Work out the finished part from the listing and answer in its coordinate system (mm). A direction names the side the tool comes from. Coordinates: 2 decimals unless noted, no trailing zeros. Order: outer loops, then holes, each group sorted by start corner. A loop starts at its lowest first (then second) coordinate and runs counter-clockwise, first axis right, second up. Notation, with made-up numbers: M 3,35.5 L 16,35.5 A8 cw 16,44.5 Z; hole C 80,57.25 d9. An arc over 180 degrees is marked long. Use a Markdown table: item, result.
from build123d import *

# Parameters (mm, degrees)
F0_W     = 5
F0_H     = 15
F1_DEPTH = 10
F3_DEPTH = 20.001
F4_W     = 10
F4_H     = 5
F5_DEPTH = 30.001


with BuildPart() as f1:
    # F0 (on Top) → F1 (new body, symmetric)
    with BuildSketch(Plane.XY):
        Polygon((0, 20), (0, 0), (20, 0), (20, 5), (25, 5), (25, 20), align=None)
        with Locations((27.5, 12.5)):
            Rectangle(F0_W, F0_H)
    extrude(amount=F1_DEPTH, both=True)

    # F2 (on Front) → F3 (cut, through all)
    with BuildSketch(Plane.XZ):
        with BuildLine():
            Line((0, 10), (0, 2.5))
            ThreePointArc((0, 2.5), (3.75, 7.916667), (10, 10))
            Line((10, 10), (0, 10))
        make_face()
        with BuildLine():
            ThreePointArc((10, -10), (3.75, -7.916667), (0, -2.5))
            Line((0, -2.5), (0, -10))
            Line((0, -10), (10, -10))
        make_face()
        Polygon((25, 10), (30, 5), (30, 10), align=None)
        Polygon((30, -10), (30, -5), (25, -10), align=None)
        with BuildLine():
            ThreePointArc((14.330127, -2.5), (14.829629, -1.294095), (15, 0))
            ThreePointArc((15, 0), (14.829629, 1.294095), (14.330127, 2.5))
            ThreePointArc((14.330127, 2.5), (10, 5), (5.669873, 2.5))
            ThreePointArc((5.669873, 2.5), (5, 0), (5.669873, -2.5))
            ThreePointArc((5.669873, -2.5), (10, -5), (14.330127, -2.5))
        make_face()
    extrude(amount=-F3_DEPTH, mode=Mode.SUBTRACT)

    # F4 (on Right) → F5 (cut, through all)
    with BuildSketch(Plane.YZ):
        with Locations((5, 0)):
            Rectangle(F4_W, F4_H)
    extrude(amount=F5_DEPTH, mode=Mode.SUBTRACT)


solid = f1.part
(1) Straight lines are drawn through the part: L1, parallel to Z at x = 24.5, y = 5.5; L2, parallel to Y at x = 25.5, z = 6.75; L3, parallel to Y at x = 17, z = 0. For each, find the intervals that lie inside material, in ascending order.
Conclusion:
| item | result |
|---|---|
| L1 | -10 to -2.5, 2.5 to 10 |
| L2 | 5 to 20 |
| L3 | 10 to 20 |
(2) A cutting plane is placed at A-A (y = 3). Determine the outline of the cut face in (x, z), then the cut area to 3 significant figures.
Conclusion:
| item | result |
|---|---|
| outline | M 0,-2.5 A10.42 ccw 10,-10 L 20,-10 L 20,-2.5 L 14.33,-2.5 A5 cw 5.67,-2.5 Z; M 0,2.5 L 5.67,2.5 A5 cw 14.33,2.5 L 20,2.5 L 20,10 L 10,10 A10.42 ccw Z |
| area | 230 mm2 |
(3) A cutting plane is placed at D-D (z = 4). Determine the outline of the cut face in (x, y), then the cut area to 3 significant figures.
Conclusion:
| item | result |
|---|---|
| outline | M 0.57,0 L 7,0 L 7,20 L 0.57,20 Z; M 13,0 L 20,0 L 20,5 L 30,5 L 30,20 L 13,20 Z |
| area | 419 mm2 |
(4) Determine the mould class of faces 4 (the flat face through (17, 10, -10)), 5 (the flat face through (22, 10, 0)), 6 (the flat face through (12, 0, 6)) for opening direction Z: pulls with the +Z half, pulls with the -Z half, needs draft (parallel to the pull), parting line crosses it, or undercut.
Conclusion:
| item | result |
|---|---|
| face 4 | pulls with the -Z half |
| face 5 | undercut |
| face 6 | needs draft |
(5) A cutting plane is placed at C-C (x = 7.5). Determine the outline of the cut face in (y, z).
Conclusion:
| item | result |
|---|---|
| outline | M 0,-9.7 L 20,-9.7 L 20,-4.33 L 0,-4.33 Z; M 0,4.33 L 20,4.33 L 20,9.7 L 0,9.7 Z |
(6) A cutting plane is placed at B-B (y = 13). Determine the outline of the cut face in (x, z).
Conclusion:
| item | result |
|---|---|
| outline | M 0,-2.5 A10.42 ccw 10,-10 L 25,-10 L 30,-5 L 30,5 L 25,10 L 10,10 A10.42 ccw 0,2.5 Z; hole M 14.33,-2.5 A5 ccw 15,0 A5 ccw 14.33,2.5 A5 ccw long Z |
(7) Which of the six approach directions +Z, -Z, +X, -X, +Y, -Y give full straight-line access (tool end or side, diameter ignored) to faces 1 (the cylindrical face through (3.825, 9.86, -7.973)), 2 (the flat face through (3, 5, 2.5)), 3 (the flat face through (24, 5, 6))?
Conclusion:
| item | result |
|---|---|
| face 1 | -Z, -X, +Y, -Y |
| face 2 | +X, -X, -Y |
| face 3 | +Z, -Z, +X, -Y |
(8) Given P1, Ø5.5, axis at x = 23, z = 0, coming from the -Y side; P2, Ø4, axis at x = 7, y = 6.5, coming from the -Z side; P3, Ø1.5, axis at y = 3, z = -3, coming from the +X side, each flat-ended and moving along its own axis, determine where each tip first touches the part or whether it passes through.
Conclusion:
| item | result |
|---|---|
| P1 | y = 5 |
| P2 | z = -9.95 |
| P3 | x = 20 |
